```python
from build123d import *

# Parameters (mm, degrees)
F0_R     = 3
F1_DEPTH = 120
F3_DEPTH = 10
F4_W     = 2
F4_H     = 2
F5_DEPTH = 3
F6_R     = 0.99999


# Not quite as in the source:
# - a fillet or chamfer is up to 0.001 mm smaller than in the source, because OpenCascade refuses the exact size


with BuildPart() as f1:
    # F0 (on Top) → F1 (new body)
    with BuildSketch(Plane.XY):
        Circle(F0_R)
    extrude(amount=F1_DEPTH)

    # F2 (on face) → F3 (cut)
    with BuildSketch(Plane(origin=(0, 0, 0), x_dir=(1, 0, 0), z_dir=(0, 0, -1))):
        with BuildLine():
            ThreePointArc((-1.2, 2.749545417), (-1.2481367635, 1.3361513276), (-2.6615308529, 1.384288091))
            ThreePointArc((-2.6615308529, 1.384288091), (-3, 0), (-2.6615308529, -1.384288091))
            ThreePointArc((-2.6615308529, -1.384288091), (-1.2481367635, -1.3361513276), (-1.2, -2.749545417))
            ThreePointArc((-1.2, -2.749545417), (0, -3), (1.2, -2.749545417))
            ThreePointArc((1.2, -2.749545417), (1.2481367635, -1.3361513276), (2.6615308529, -1.384288091))
            ThreePointArc((2.6615308529, -1.384288091), (2.9141544707, -0.7125333119), (3, 0))
            ThreePointArc((3, 0), (2.9141544707, 0.7125333119), (2.6615308529, 1.384288091))
            ThreePointArc((2.6615308529, 1.384288091), (1.2481367635, 1.3361513276), (1.2, 2.749545417))
            ThreePointArc((1.2, 2.749545417), (0, 3), (-1.2, 2.749545417))
        make_face()
    extrude(amount=-F3_DEPTH, mode=Mode.SUBTRACT)

    # F4 (on face) → F5 (join)
    with BuildSketch(Plane(origin=(0, 0, 10), x_dir=(1, 0, 0), z_dir=(0, 0, -1))):
        Rectangle(F4_W, F4_H)
    extrude(amount=F5_DEPTH)

    # F6 (radius 1 in the source; OpenCascade refuses exactly that, so slightly less here)
    f6_edges = [f1.edges().sort_by_distance(p)[0] for p in [
        (0, -1, 7),
        (-1, 0, 7),
        (0, 1, 7),
        (1, 0, 7),
        (1, -1, 8.5),
        (1, 1, 8.5),
        (-1, -1, 8.5),
        (-1, 1, 8.5),
    ]]
    fillet(f6_edges, radius=F6_R)


solid = f1.part
```
Model file for the job. Use its own axes, mm. Coordinates: 2 decimals unless noted, no trailing zeros. Loops run counter-clockwise (first coordinate to the right, second up) from the corner with the lowest first, then second, coordinate; pieces in that order, holes last. Notation, with made-up numbers: M -15,-27.5 L 26,-27.5 A27 ccw 26,-7.5 Z; hole C 67,31.25 d11. An arc over 180 degrees is marked long. Use CSV: the item, a comma, the result in double quotes. Start each with the question number.
1. Probe probe 1 along Z at (x, y) = (1.95, 0.8); probe 2 along X at (y, z) = (2.55, 9); probe 3 along X at (y, z) = (-0.2, 9.5). List the from-to ranges inside material, lowest first. Write a range as [from, to].
2. Flat gauge pins, fed straight in: pin 1 (2 mm diameter, centred on x = -1.5, z = 60, fed in from +Y); pin 2 (1 mm diameter, centred on y = -2, z = 89, fed in from +X). Where does each tip first touch, or does it go through?
3. Two-plate mould, pull along Y, no slides. Class faces 1 (the flat face through (0, 0, 120)), 2 (the flat face through (-1, -1, 10)), 3 (the cylindrical face through (-3, 0, 59)): pulls with the +Y half, pulls with the -Y half, needs draft (parallel to the pull), parting line crosses it, or undercut.
4. Band-saw the part on A-A, the plane z = 85.5. List the corners of the cut face in (x, y), then the cut area to 3 significant figures.
Entries:
1,probe 1,"z = [10, 120]"
1,probe 2,"x = [-1.58, -1.06], [1.06, 1.58]"
1,probe 3,"x = [-0.98, 0.98]"
2,pin 1,"stops at y = 2.96"
2,pin 2,"stops at x = 2.6"
3,face 1,"needs draft"
3,face 2,"undercut"
3,face 3,"parting line crosses it"
4,outline,"C 0,0 d6"
4,area,"28.3 mm2"
